from build123d import *

# Parameters (mm, degrees)
CHAMFER1_SIZE = 0.319532


with BuildPart() as part:
    # Sketch2 → Revolve1 (revolve)
    with BuildSketch(Plane(origin=(0, 0, 0), x_dir=(0, 0, -1), z_dir=(1, 0, 0)), mode=Mode.PRIVATE) as revolve1_sk:
        with BuildLine():
            Line((0, 0), (0, 1.5875))
            ThreePointArc((0, 1.5875), (3.077438862, 2.771171998), (6.35, 3.17373))
            Line((6.35, 3.17373), (8.3058, 3.17373))
            Line((8.3058, 3.17373), (8.3058, 3.0150435))
            Line((8.3058, 3.0150435), (9.525, 3.0150435))
            Line((9.525, 3.0150435), (9.525, 3.556))
            Line((9.525, 3.556), (10.3378, 3.556))
            Line((10.3378, 3.556), (10.3378, 3.0150435))
            Line((10.3378, 3.0150435), (11.557, 3.0150435))
            Line((11.557, 3.0150435), (11.557, 3.19532))
            Line((11.557, 3.19532), (23.0378, 3.19532))
            Line((23.0378, 3.19532), (23.0378, 0))
            Line((23.0378, 0), (0, 0))
        make_face()
    revolve(revolve1_sk.sketch.rotate(Axis((0, 0, 0), (0, 0, 1)), 90), axis=Axis((0, 0, 0), (0, 0, 1)))

    # Chamfer1
    chamfer1_edges = [part.edges().sort_by_distance(p)[0] for p in [
        (3.19532, 0, -23.0378),
    ]]
    chamfer(chamfer1_edges, length=CHAMFER1_SIZE)


solid = part.part
For this review, take the finished solid that the model builds, in its own axes (mm). A direction names the side the tool comes from. Round coordinates to 2 decimals unless told otherwise and drop trailing zeros. Write each loop counter-clockwise with the first axis right and the second up, starting at its lowest first coordinate (ties: lowest second). Pieces come first, ordered by that corner, then holes. Notation, with made-up numbers: (89, 69) - (111, 69) arc R20 cw to (111, 93) - close; hole circle Ø7 at (5.5, 51). An arc over 180 degrees is marked (long way). Use a Markdown table: item, result.
Q1. Machinability: for faces 5 (the cylindrical face through (0.416, -3.168, -17.216)), 6 (the cylindrical face through (0.688, 3.098, -7.342)), 7 (the cylindrical face through (0.39, -2.99, -8.92)), which of the approach directions +Z, -Z, +X, -X, +Y, -Y give a long, thin tool a straight path to every point of the face, cutting with its end or side? Answer none if there is none.
Derived:
| item | result |
|---|---|
| face 5 | -Z |
| face 6 | +Z |
| face 7 | none |
Q2. Wall thickness on line 1 along Z through (x, y) = (-0.5, 3.25) (3 decimals); line 2 along Y through (x, z) = (0.5, -17.5); line 3 along X through (y, z) = (-1.5, -3.75): over which ranges is each line inside the solid? List them lowest first.
Derived:
| item | result |
|---|---|
| line 1 | z = -10.338 to -9.525 |
| line 2 | y = -3.16 to 3.16 |
| line 3 | x = -2.51 to 2.51 |
Q3. The part is to be moulded in two halves that separate along Z. For faces 1 (the cylindrical face through (0.77, 3.47, -9.94)), 2 (the flat face through (0, 0, -23.038)), 3 (the cylindrical face through (0.39, -2.99, -10.96)), 4 (the flat face through (0, 0, 0)), say which applies: pulls with the +Z half, pulls with the -Z half, needs draft (parallel to the pull), parting line crosses it, or undercut.
Derived:
| item | result |
|---|---|
| face 1 | needs draft |
| face 2 | pulls with the -Z half |
| face 3 | undercut |
| face 4 | pulls with the +Z half |
Q4. We need section B-B (z = -11.25). Give the boundary of the cut face in (x, y).
Derived:
| item | result |
|---|---|
| outline | circle Ø6.03 at (0, 0) |
Q5. Clearance check with flat-ended pins moving along their axes: pin 1 (4 mm diameter, centred on x = 1.5, y = -2.5, fed in from +Z); pin 2 (4 mm diameter, centred on y = 2, z = -6.5, fed in from +X). State where each tip first meets the part, or that it passes through.
Derived:
| item | result |
|---|---|
| pin 1 | stops at z = 0 |
| pin 2 | stops at x = 3.17 |
Q6. We need section A-A (z = -15.5). Give the boundary of the cut face in (x, y).
Derived:
| item | result |
|---|---|
| outline | circle Ø6.39 at (0, 0) |
